from build123d import *

# Parameters (mm, degrees)
F1_DEPTH      = 1
F2_R          = 0.8
F3_DEPTH      = 25
F3_DEPTH_BACK = 25
F5_START      = -1.001
F5_DEPTH      = 23.999
F6_R          = 1
F8_DEPTH      = 0.6
F9_R          = 0.5
F10_R         = 1.3
F11_DEPTH     = 0.4


with BuildPart() as f1:
    # F0 (on Front) → F1 (new body)
    with BuildSketch(Plane.XZ):
        Polygon((3.5355339059, 6.123724357), (0, 0), (16.5950652481, -28.7434961647), (20.7974290086, -28.7434961647), (8, 0), (8, 7.3199744415), align=None)
    extrude(amount=F1_DEPTH)

    # F2 (on face) → F3 (cut, two sides)
    with BuildSketch(Plane.XZ.offset(1)) as f3_sk:
        with Locations((3, 0)):
            Circle(F2_R)
        with Locations((6, 0)):
            Circle(F2_R)
    extrude(amount=-F3_DEPTH, mode=Mode.SUBTRACT)
    extrude(f3_sk.sketch, amount=F3_DEPTH_BACK, mode=Mode.SUBTRACT)

    # F4 (on face) → F5 (cut)
    with BuildSketch(Plane.XZ.offset(1).offset(F5_START)):
        Polygon((8, -3.5337661579), (3.9760127691, -3.5337661579), (16.3063901135, -26.2434961647), (18.5897210168, -26.2434961647), align=None)
    extrude(amount=-F5_DEPTH, mode=Mode.SUBTRACT)

    # F6
    f6_edges = [f1.edges().sort_by_distance(p)[0] for p in [
        (16.595065, -0.5, -28.743496),
        (20.797429, -0.5, -28.743496),
        (3.535534, -0.5, 6.123724),
        (8, -0.5, 7.319974),
    ]]
    fillet(f6_edges, radius=F6_R)

    # F7 (on face) → F8 (cut)
    with BuildSketch(Plane.XZ.offset(1)):
        Polygon((2.3094010768, 2), (7, 2), (7, 6.0167490687), (4.1944525285, 5.2650048894), align=None)
        Polygon((17.1724155173, -27.7434961647), (19.2575640448, -27.7434961647), (7.9293896977, -2.3), (2.4826061575, -2.3), align=None)
    extrude(amount=-F8_DEPTH, mode=Mode.SUBTRACT)

    # F9
    f9_edges = [f1.edges().sort_by_distance(p)[0] for p in [
        (2.309401, -0.7, 2),
        (7, -0.7, 2),
        (7, -0.7, 6.016749),
        (4.194453, -0.7, 5.265005),
        (7.92939, -0.7, -2.3),
        (2.482606, -0.7, -2.3),
        (19.257564, -0.7, -27.743496),
        (17.172416, -0.7, -27.743496),
    ]]
    fillet(f9_edges, radius=F9_R)

    # F10 (on face) → F11 (cut)
    with BuildSketch(Plane.XZ.offset(1)):
        with Locations((3, 0)):
            Circle(F10_R)
        with Locations((6, 0)):
            Circle(F10_R)
    extrude(amount=-F11_DEPTH, mode=Mode.SUBTRACT)


solid = f1.part
Read the model definition and answer for the solid it produces. Units are mm, in the model's axes. A direction names the side the tool comes from. Give positions to 0.01 mm unless a question says otherwise; leave off trailing zeros. Loops run counter-clockwise (first coordinate to the right, second up) from the corner with the lowest first, then second, coordinate; pieces in that order, holes last. Notation, with made-up numbers: (70.5, 63) -> (99.5, 63) arc R27 cw to (99.5, 84) -> close; hole circle Ø5 at (37.5, -24). An arc over 180 degrees is marked (long way). Use a Markdown table: item, result.
Q1. Section D-D, the plane x = 9.5 is taken. Determine the outline of the cut face in (y, z).
Solved:
| item | result |
|---|---|
| outline | (-1, -16.45) -> (0, -16.45) -> (0, -3.37) -> (-1, -3.37) -> (-1, -5.83) -> (-0.4, -5.83) -> (-0.4, -14.45) -> (-1, -14.45) -> close |
Q2. Section C-C, the plane z = -10 is taken. Determine the outline of the cut face in (x, y).
Solved:
| item | result |
|---|---|
| outline | (5.77, -1) -> (6.93, -1) -> (6.93, -0.4) -> (11.36, -0.4) -> (11.36, -1) -> (12.45, -1) -> (12.45, 0) -> (5.77, 0) -> close |
Q3. Determine the mould class of faces 3 (the face through (1.688, -0.493, 2.923)), 4 (the face through (8.039, -0.493, -13.924)), 5 (the face through (8, -0.5, 3)), 6 (the face through (11, -0.4, -13)) for opening direction Z: pulls with the +Z half, pulls with the -Z half, needs draft (parallel to the pull), parting line crosses it, or undercut.
Solved:
| item | result |
|---|---|
| face 3 | pulls with the +Z half |
| face 4 | pulls with the -Z half |
| face 5 | needs draft |
| face 6 | undercut |
Q4. Find the intervals of material crossed by line 1 along Y through (x, z) = (8, -7.5); line 2 along Z through (x, y) = (3, -0.65); line 3 along X through (y, z) = (-0.85, -24), in increasing order.
Solved:
| item | result |
|---|---|
| line 1 | y = -0.4 to 0 |
| line 2 | z = -5.2 to -3.2, -2.44 to -1.3, 1.3 to 2.03, 3.2 to 5.2 |
| line 3 | x = 13.86 to 15.01, 17.59 to 18.69 |
Q5. A tool of negligible diameter and unlimited length cuts with its end or side. For faces 1 (the face through (5, -0.4, 4)), 2 (the face through (9, 0, -9)), from which of +Z, -Z, +X, -X, +Y, -Y can it reach the whole face along a straight path? Write none if from no direction.
Solved:
| item | result |
|---|---|
| face 1 | -Y |
| face 2 | +Z, -Z, +X, -X, +Y |
Q6. Each of these flat-tipped pins is pushed along its axis until it touches: pin 1 (2.5 mm diameter, centred on x = 3, z = 0, fed in from -Y); pin 2 (0.5 mm diameter, centred on x = 4.5, y = -1, fed in from +Z); pin 3 (1.9 mm diameter, centred on x = 5, z = 4, fed in from -Y). Where does it stop, or does it pass through?
Solved:
| item | result |
|---|---|
| pin 1 | stops at y = -0.6 |
| pin 2 | stops at z = 6.45 |
| pin 3 | stops at y = -0.4 |
Q7. Section A-A, the plane y = -0.85 is taken. Count the separate pieces of the cut face and the enclosed holes in it, then the cut area to 3 significant figures.
Solved:
| item | result |
|---|---|
| separate pieces | 1 |
| enclosed holes | 4 |
| area | 96.1 mm^2 |
Q8. Section B-B, the plane x = 6 is taken. Determine the outline of the cut face in (y, z), then the cut area to 3 significant figures.
Solved:
| item | result |
|---|---|
| outline | (-1, -10.39) -> (0, -10.39) -> (0, -0.8) -> (-0.6, -0.8) -> (-0.6, -1.3) -> (-1, -1.3) -> (-1, -2.3) -> (-0.4, -2.3) -> (-0.4, -8.39) -> (-1, -8.39) -> close; (-1, 1.3) -> (-0.6, 1.3) -> (-0.6, 0.8) -> (0, 0.8) -> (0, 6.78) -> (-1, 6.78) -> (-1, 5.75) -> (-0.4, 5.75) -> (-0.4, 2) -> (-1, 2) -> close |
| area | 9.27 mm^2 |
